Model file for the job. Use its own axes, mm. Face numbers are marked on the shaded views. Coordinates: 2 decimals unless noted, no trailing zeros. Order: outer loops, then holes, each group sorted by start corner. A loop starts at its lowest first (then second) coordinate and runs counter-clockwise, first axis right, second up. Notation, with made-up numbers: (-19, -7.5) -> (20, -7.5) arc R9 cw to (20, 7.5) -> close; hole circle Ø6 at (31, 3.25). An arc over 180 degrees is marked (long way). Write item = value, one per line. Start each with the question number.
Q1. Cut at B-B, the plane z = 0. List the corners of the cut face in (x, y), plus the area to 3 significant figures.
Q2. Cut at C-C, the plane z = 13.5. List the corners of the cut face in (x, y).
Q3. Cut at A-A, the plane x = 0. List the corners of the cut face in (y, z).
Q4. Mould opens along X. For the marked faces 1, 2 and 3 say: +X half, -X half, draft (parallel to the pull), parting line (faces both ways), or undercut.
Q5. Wall check: line 1 (X direction, y = 1.75, z = -14); line 2 (Z direction, x = 20.5, y = 2); line 3 (Z direction, x = -15, y = 4). Give the ranges that are in metal, low to high. Write a range as from..to.
Q6. Cut at D-D, the plane y = 4.75. Give the number of separate pieces and of enclosed holes in the cut face, plus the area to 3 significant figures.
Q7. Flat gauge pins, fed straight in: pin 1 (2.5 mm diameter, centred on x = 13.96, z = -19.21, fed in from +Y); pin 2 (4 mm diameter, centred on x = 19.21, z = -13.96, fed in from +Y); pin 3 (1 mm diameter, centred on y = 4.5, z = -17.5, fed in from -X); pin 4 (1.5 mm diameter, centred on x = 2, z = -19.5, fed in from +Y). Where does each tip first touch, or does it go through?
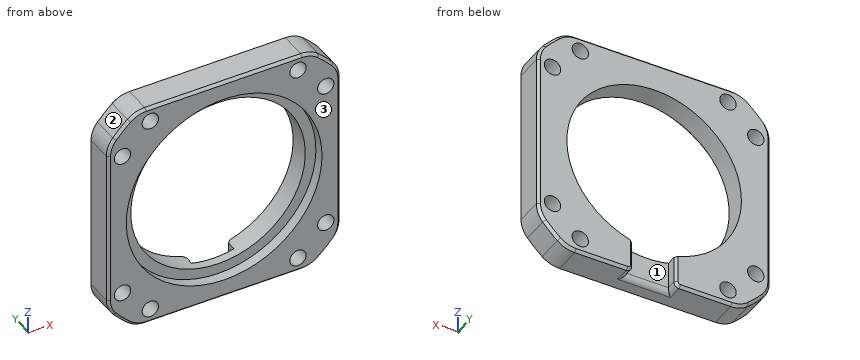
from build123d import *

# Parameters (mm, degrees)
EXTRUDE_1_DEPTH      = 6
SKETCH_2_R           = 10.5
CUT_EXTRUDE_1_DEPTH  = 10
SKETCH_3_R           = 1.55
CUT_EXTRUDE_2_DEPTH  = 10
SKETCH_7_W           = 16
SKETCH_7_H           = 44.832254491
CUT_EXTRUDE_4_DEPTH  = 10
FILLET_1_R           = 3
FILLET_2_R           = 5
EXTRUDE_START        = -6
EXTRUDE_2_DEPTH      = 6
SKETCH_9_R           = 9.75
CUT_EXTRUDE_5_DEPTH  = 32.685959036
SKETCH_10_R          = 13
CUT_EXTRUDE_6_DEPTH  = 2
SKETCH_11_W          = 8
SKETCH_11_H          = 16
CUT_EXTRUDE_7_DEPTH  = 2.3
FILLET_3_R           = 1
EXTRUDE_3_DEPTH      = 6
SKETCH_13_W          = 8
SKETCH_13_H          = 3
CUT_EXTRUDE_8_DEPTH  = 2.3
FILLET_4_R           = 1
CHAMFER_1_SIZE       = 0.5
EXTRUDE_START_2      = 3
SKETCH_14_R          = 15
SKETCH_14_R_2        = 13
EXTRUDE_4_DEPTH      = 3
CHAMFER_2_SIZE       = 0.5
SKETCH_15_R          = 17.000673468
CUT_EXTRUDE_9_DEPTH  = 23
SKETCH_17_R          = 18.5
CUT_EXTRUDE_11_DEPTH = 2
SKETCH_18_R          = 16.5
CUT_EXTRUDE_12_DEPTH = 14


with BuildPart() as part:
    # 草图1 → 凸台-拉伸1 (new body)
    with BuildSketch(Plane(origin=(0, 0, 0), x_dir=(1, 0, 0), z_dir=(0, 1, 0))):
        with BuildLine():
            Line((-16.5, 22), (16.5, 22))
            ThreePointArc((16.5, 22), (19.445436483, 19.445436483), (22, 16.5))
            Line((22, 16.5), (22, -16.5))
            ThreePointArc((22, -16.5), (19.445436483, -19.445436483), (16.5, -22))
            Line((16.5, -22), (-16.5, -22))
            ThreePointArc((-16.5, -22), (-19.445436483, -19.445436483), (-22, -16.5))
            Line((-22, -16.5), (-22, 16.5))
            ThreePointArc((-22, 16.5), (-19.445436483, 19.445436483), (-16.5, 22))
        make_face()
    extrude(amount=EXTRUDE_1_DEPTH)

    # 草图2 → 切除-拉伸1 (cut)
    with BuildSketch(Plane(origin=(0, 6, 0), x_dir=(1, 0, 0), z_dir=(0, 1, 0))):
        with Locations(Location((0, 0, 0), (0, 0, 270))):
            Circle(SKETCH_2_R)
    extrude(amount=-CUT_EXTRUDE_1_DEPTH, mode=Mode.SUBTRACT)

    # 草图3 → 切除-拉伸2 (cut)
    with BuildSketch(Plane(origin=(0, 6, 0), x_dir=(1, 0, 0), z_dir=(0, 1, 0))):
        with Locations(Location((-19.214153616, 13.959899742, 0), (0, 0, 270))):
            Circle(SKETCH_3_R)
        with Locations(Location((-13.959899742, 19.214153616, 0), (0, 0, 270))):
            Circle(SKETCH_3_R)
        with Locations(Location((19.214153616, 13.959899742, 0), (0, 0, 270))):
            Circle(SKETCH_3_R)
        with Locations(Location((13.959899742, 19.214153616, 0), (0, 0, 270))):
            Circle(SKETCH_3_R)
        with Locations(Location((19.214153616, -13.959899742, 0), (0, 0, 270))):
            Circle(SKETCH_3_R)
        with Locations(Location((13.959899742, -19.214153616, 0), (0, 0, 270))):
            Circle(SKETCH_3_R)
        with Locations(Location((-19.214153616, -13.959899742, 0), (0, 0, 270))):
            Circle(SKETCH_3_R)
        with Locations(Location((-13.959899742, -19.214153616, 0), (0, 0, 270))):
            Circle(SKETCH_3_R)
    extrude(amount=-CUT_EXTRUDE_2_DEPTH, mode=Mode.SUBTRACT)

    # 草图7 → 切除-拉伸4 (cut)
    with BuildSketch(Plane(origin=(0, 6, 0), x_dir=(1, 0, 0), z_dir=(0, 1, 0))):
        with Locations((0, 26.514900262)):
            Rectangle(SKETCH_7_W, SKETCH_7_H)
    extrude(amount=-CUT_EXTRUDE_4_DEPTH, mode=Mode.SUBTRACT)

    # 圆角1
    fillet_1_edges = [part.edges().sort_by_distance(p)[0] for p in [
        (-8, 3, -22),
        (8, 3, -22),
    ]]
    fillet(fillet_1_edges, radius=FILLET_1_R)

    # 圆角2
    fillet_2_edges = [part.edges().sort_by_distance(p)[0] for p in [
        (-16.5, 3, -22),
        (16.5, 3, -22),
        (22, 3, -16.5),
        (22, 3, 16.5),
        (16.5, 3, 22),
        (-16.5, 3, 22),
        (-22, 3, 16.5),
        (-22, 3, -16.5),
    ]]
    fillet(fillet_2_edges, radius=FILLET_2_R)

    # 草图8 → 凸台-拉伸2 (add)
    with BuildSketch(Plane.XZ.offset(EXTRUDE_START)):
        with BuildLine():
            Line((8, -6.800735254), (8, -19))
            Line((8, -19), (-8, -19))
            Line((-8, -19), (-8, -6.800735254))
            ThreePointArc((-8, -6.800735254), (0, 10.5), (8, -6.800735254))
        make_face()
    extrude(amount=EXTRUDE_2_DEPTH)

    # 草图9 → 切除-拉伸5 (cut, through all)
    with BuildSketch(Plane.XZ):
        with Locations(Location((0, 0, 0), (0, 0, 270))):
            Circle(SKETCH_9_R)
    extrude(amount=-CUT_EXTRUDE_5_DEPTH, mode=Mode.SUBTRACT)

    # 草图10 → 切除-拉伸6 (cut)
    with BuildSketch(Plane.XZ):
        with Locations(Location((0, 0, 0), (0, 0, 270))):
            Circle(SKETCH_10_R)
    extrude(amount=-CUT_EXTRUDE_6_DEPTH, mode=Mode.SUBTRACT)

    # 草图11 → 切除-拉伸7 (cut)
    with BuildSketch(Plane(origin=(0, 6, 0), x_dir=(1, 0, 0), z_dir=(0, 1, 0))):
        with Locations((0, 16.891709622)):
            Rectangle(SKETCH_11_W, SKETCH_11_H)
    extrude(amount=-CUT_EXTRUDE_7_DEPTH, mode=Mode.SUBTRACT)

    # 圆角3
    fillet_3_edges = [part.edges().sort_by_distance(p)[0] for p in [
        (4, 4.85, -8.891709622),
        (-4, 4.85, -8.891709622),
        (2.045523305, 3.7, -9.533012871),
    ]]
    fillet(fillet_3_edges, radius=FILLET_3_R)

    # 草图12 → 凸台-拉伸3 (add)
    with BuildSketch(Plane.XZ):
        with BuildLine():
            Line((-11, -22), (11, -22))
            ThreePointArc((11, -22), (8.878679656, -21.121320344), (8, -19))
            Line((8, -19), (-8, -19))
            ThreePointArc((-8, -19), (-8.878679656, -21.121320344), (-11, -22))
        make_face()
    extrude(amount=-EXTRUDE_3_DEPTH)

    # 草图13 → 切除-拉伸8 (cut)
    with BuildSketch(Plane(origin=(0, 6, 0), x_dir=(1, 0, 0), z_dir=(0, 1, 0))):
        with Locations((0, 20.5)):
            Rectangle(SKETCH_13_W, SKETCH_13_H)
    extrude(amount=-CUT_EXTRUDE_8_DEPTH, mode=Mode.SUBTRACT)

    # 圆角4
    fillet_4_edges = [part.edges().sort_by_distance(p)[0] for p in [
        (0, 3.7, -22),
        (-4, 4.85, -22),
        (4, 4.85, -22),
    ]]
    fillet(fillet_4_edges, radius=FILLET_4_R)

    # 倒角1
    chamfer_1_edges = [part.edges().sort_by_distance(p)[0] for p in [
        (9.869701486, 6, -22),
        (0, 0, -22),
        (19.445436483, 0, 19.445436483),
        (19.445436483, 6, 19.445436483),
        (19.445436483, 0, -19.445436483),
        (22, 0, 0),
        (0, 0, 22),
        (-19.445436483, 0, 19.445436483),
        (-22, 0, 0),
        (-19.445436483, 0, -19.445436483),
        (-16.48741772, 0, -21.684489774),
        (-21.684489774, 0, -16.48741772),
        (-21.684489774, 0, 16.48741772),
        (-16.48741772, 0, 21.684489774),
        (16.48741772, 0, -21.684489774),
        (21.684489774, 0, -16.48741772),
        (21.684489774, 0, 16.48741772),
        (16.48741772, 0, 21.684489774),
        (0, 6, 22),
        (-19.445436483, 6, -19.445436483),
        (-22, 6, 0),
        (-19.445436483, 6, 19.445436483),
        (22, 6, 0),
        (19.445436483, 6, -19.445436483),
        (-16.48741772, 6, -21.684489774),
        (-21.684489774, 6, -16.48741772),
        (-21.684489774, 6, 16.48741772),
        (-16.48741772, 6, 21.684489774),
        (16.48741772, 6, -21.684489774),
        (21.684489774, 6, -16.48741772),
        (21.684489774, 6, 16.48741772),
        (16.48741772, 6, 21.684489774),
        (0, 6, 9.75),
        (4, 6, -15.258216578),
        (4.144103897, 6, -8.999285342),
        (-4.144103897, 6, -8.999285342),
        (-4, 6, -15.258216578),
        (-9.869701486, 6, -22),
        (4.292893219, 6, -21.707106781),
        (-4.292893219, 6, -21.707106781),
    ]]
    chamfer(chamfer_1_edges, length=CHAMFER_1_SIZE)

    # 草图14 → 凸台-拉伸4 (add)
    with BuildSketch(Plane.XZ.offset(EXTRUDE_START_2)):
        with Locations(Location((0, 0, 0), (0, 0, 90))):
            Circle(SKETCH_14_R)
        with Locations(Location((0, 0, 0), (0, 0, 270))):
            Circle(SKETCH_14_R_2, mode=Mode.SUBTRACT)
    extrude(amount=-EXTRUDE_4_DEPTH)

    # 倒角2
    chamfer_2_edges = [part.edges().sort_by_distance(p)[0] for p in [
        (0, -3, -15),
        (0, -3, 13),
    ]]
    chamfer(chamfer_2_edges, length=CHAMFER_2_SIZE)

    # 草图15 → 切除-拉伸9 (cut)
    with BuildSketch(Plane.XZ):
        Circle(SKETCH_15_R)
    extrude(amount=CUT_EXTRUDE_9_DEPTH, mode=Mode.SUBTRACT)

    # 草图17 → 切除-拉伸11 (cut)
    with BuildSketch(Plane.XZ):
        with Locations(Location((0, 0, 0), (0, 0, 270))):
            Circle(SKETCH_17_R)
    extrude(amount=-CUT_EXTRUDE_11_DEPTH, mode=Mode.SUBTRACT)

    # 草图18 → 切除-拉伸12 (cut)
    with BuildSketch(Plane.XZ.offset(-2)):
        with Locations(Location((0, 0, 0), (0, 0, 270))):
            Circle(SKETCH_18_R)
    extrude(amount=-CUT_EXTRUDE_12_DEPTH, mode=Mode.SUBTRACT)


solid = part.part
Here are the results:
q1.outline = (-22, 0.5) -> (-21.5, 0) -> (-18.5, 0) -> (-18.5, 2) -> (-16.5, 2) -> (-16.5, 6) -> (-21.5, 6) -> (-22, 5.5) -> close; (16.5, 2) -> (18.5, 2) -> (18.5, 0) -> (21.5, 0) -> (22, 0.5) -> (22, 5.5) -> (21.5, 6) -> (16.5, 6) -> close
q1.area = 57.5 mm²
q2.outline = (-22, 0.5) -> (-21.5, 0) -> (-20.69, 0) -> (-20.69, 6) -> (-21.5, 6) -> (-22, 5.5) -> close; (-17.73, 0) -> (-12.65, 0) -> (-12.65, 2) -> (-9.49, 2) -> (-9.49, 6) -> (-17.73, 6) -> close; (9.49, 2) -> (12.65, 2) -> (12.65, 0) -> (17.73, 0) -> (17.73, 6) -> (9.49, 6) -> close; (20.69, 0) -> (21.5, 0) -> (22, 0.5) -> (22, 5.5) -> (21.5, 6) -> (20.69, 6) -> close
q3.outline = (0, -21.5) -> (0.5, -22) -> (2.7, -22) arc R1 ccw to (3.7, -21) -> (3.7, -16.5) -> (2, -16.5) -> (2, -18.5) -> (0, -18.5) -> close; (0, 18.5) -> (2, 18.5) -> (2, 16.5) -> (6, 16.5) -> (6, 21.5) -> (5.5, 22) -> (0.5, 22) -> (0, 21.5) -> close
q4.face_1 = undercut
q4.face_2 = -X half
q4.face_3 = draft
q5.line_1 = -22..-20.76, -17.66..-12.09, 12.09..17.66, 20.76..22
q5.line_2 = -18.33..-14.83, -13.09..13.09, 14.83..18.33
q5.line_3 = -21.99..-20.36, -18.06..-6.87, 6.87..18.06, 20.36..21.99
q6.separate_pieces = 1
q6.enclosed_holes = 8
q6.area = 917 mm²
q7.pin_1 = through
q7.pin_2 = 6
q7.pin_3 = -21.46
q7.pin_4 = 3.7
